The figure shows three views and two pictorial views of one solid part (mm, origin at its lowest corner). Answer the questions. Round coordinates to 2 decimals unless told otherwise and drop trailing zeros. Order: outer loops, then holes, each group sorted by start corner. A loop starts at its lowest first (then second) coordinate and runs counter-clockwise, first axis right, second up. Notation, with made-up numbers: (74, 24.5) - (113, 24.5) arc R24 cw to (113, 49.5) - close; hole circle Ø6 at (77, 5). An arc over 180 degrees is marked (long way). Answer in a Markdown table with one row per item.
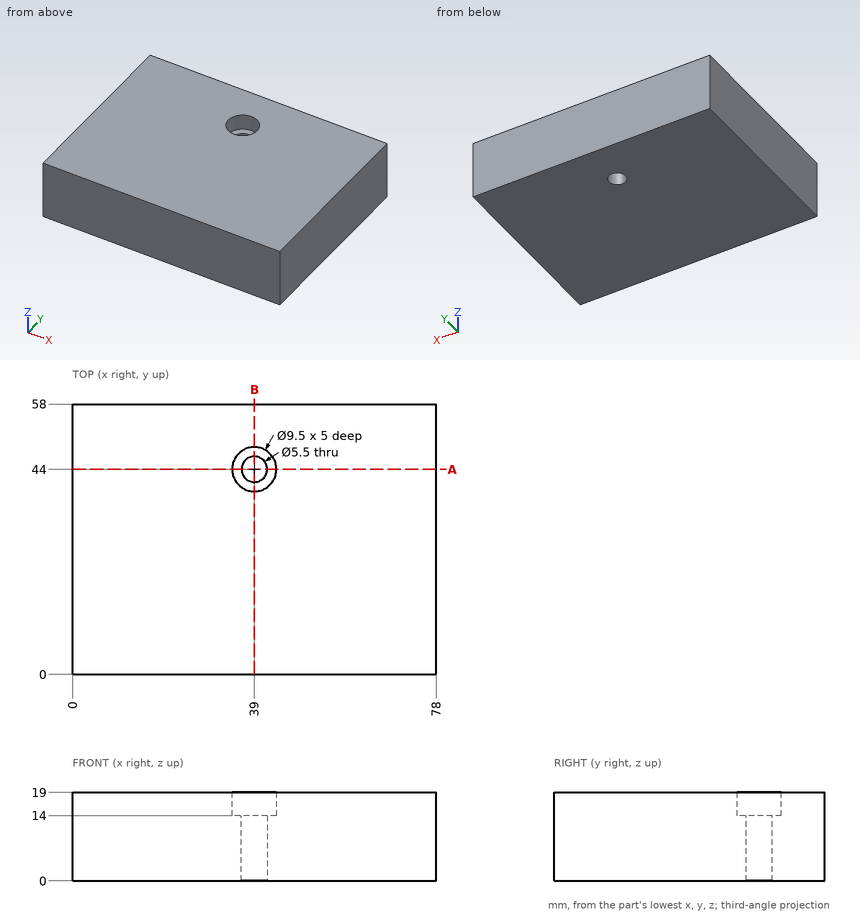
1) This flat-tipped pin is pushed along its axis until it touches: pin 1 (8.5 mm diameter, centred on x = 39, y = 44, fed in from +Z). Where does it stop, or does it pass through?
Filled in:
| item | result |
|---|---|
| pin 1 | stops at z = 14 |
2) Find section B-B, the plane x = 39. Give the vertices of the cut face in (y, z).
Filled in:
| item | result |
|---|---|
| outline | (0, 0) - (41.25, 0) - (41.25, 14) - (39.25, 14) - (39.25, 19) - (0, 19) - close; (46.75, 0) - (58, 0) - (58, 19) - (48.75, 19) - (48.75, 14) - (46.75, 14) - close |
3) Find the intervals of material crossed by probe 1 along Y at (x, z) = (39, 16.4); probe 2 along Y at (x, z) = (39, 4); probe 3 along X at (y, z) = (43, 15), in increasing order. Write a range as from..to.
Filled in:
| item | result |
|---|---|
| probe 1 | y = 0..39.25, 48.75..58 |
| probe 2 | y = 0..41.25, 46.75..58 |
| probe 3 | x = 0..34.36, 43.64..78 |
4) Find section A-A, the plane y = 44. Give the vertices of the cut face in (x, z), then the cut area to 3 significant figures.
Filled in:
| item | result |
|---|---|
| outline | (0, 0) - (36.25, 0) - (36.25, 14) - (34.25, 14) - (34.25, 19) - (0, 19) - close; (41.75, 0) - (78, 0) - (78, 19) - (43.75, 19) - (43.75, 14) - (41.75, 14) - close |
| area | 1,360 mm^2 |
